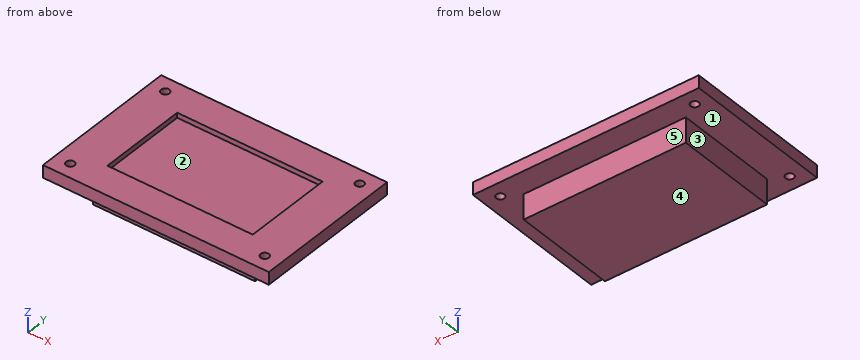
from build123d import *

# Parameters (mm, degrees)
F0_W     = 115
F0_H     = 76.2
F1_DEPTH = 6.35
F2_W     = 82.55
F2_H     = 52.3875
F3_DEPTH = 12.7
F4_W     = 74
F4_H     = 45
F5_DEPTH = 2.54
F7_D     = 4.1656


with BuildPart() as f1:
    # F0 (on Top) → F1 (new body)
    with BuildSketch(Plane.XY):
        with Locations((4.230735, 2.938756)):
            Rectangle(F0_W, F0_H)
    extrude(amount=F1_DEPTH)

    # F2 (on face) → F3 (join)
    with BuildSketch(Plane(origin=(0, 0, 0), x_dir=(1, 0, 0), z_dir=(0, 0, -1))):
        with Locations((4.225135, -2.716506)):
            Rectangle(F2_W, F2_H)
    extrude(amount=F3_DEPTH)

    # F4 (on face) → F5 (cut)
    with BuildSketch(Plane.XY.offset(6.35)):
        with Locations((4.228535, 2.943156)):
            Rectangle(F4_W, F4_H)
    extrude(amount=-F5_DEPTH, mode=Mode.SUBTRACT)

    # F7 (through all)
    with Locations(Plane.XY.offset(6.35)):
        with Locations((-45.269265, 33.538756), (53.730735, 33.538756), (53.730735, -27.668244), (-45.269265, -27.668244)):
            Hole(F7_D / 2)


solid = f1.part
For this review, take the finished solid that the model builds, in its own axes (mm). Face numbers are marked on the shaded views. A direction names the side the tool comes from. Coordinates: 2 decimals unless noted, no trailing zeros. Loops run counter-clockwise (first coordinate to the right, second up) from the corner with the lowest first, then second, coordinate; pieces in that order, holes last. Notation, with made-up numbers: (71, -25) - (111, -25) arc R24 cw to (111, -6) - close; hole circle Ø9 at (-33.5, -9). An arc over 180 degrees is marked (long way). Return JSON: item names as keys, results as strings.
Item 1: Take a section at C-C (z = -6.75). Give the boundary of the cut face in (x, y).
Determined:
{"outline": "(-37.05, -23.48) - (45.5, -23.48) - (45.5, 28.91) - (-37.05, 28.91) - close"}
Item 2: Take a section at B-B (x = 11). Give the boundary of the cut face in (y, z).
Determined:
{"outline": "(-35.16, 0) - (-23.48, 0) - (-23.48, -12.7) - (28.91, -12.7) - (28.91, 0) - (41.04, 0) - (41.04, 6.35) - (25.44, 6.35) - (25.44, 3.81) - (-19.56, 3.81) - (-19.56, 6.35) - (-35.16, 6.35) - close"}
Item 3: For the marked faces 4 and 5, list the 3-axis set-ups (+Z, -Z, +X, -X, +Y, -Y) from which the entire face can be reached by the end or side of a thin tool; tool diameter is ignored.
Determined:
{"face 4": "-Z, +X, -X, +Y, -Y", "face 5": "-Z, +X, -X, +Y"}
Item 4: Mouldability with a two-part tool opening along X and no side actions: class the marked faces 1, 2 and 3 as pulls with the +X half, pulls with the -X half, needs draft (parallel to the pull), parting line crosses it, or undercut.
Determined:
{"face 1": "needs draft", "face 2": "undercut", "face 3": "pulls with the -X half"}
Item 5: For line 1 (X direction, y = -15.5, z = 5.75); line 2 (Z direction, x = 40.5, y = 35.5); line 3 (Y direction, x = -1.5, z = -5), list the stretches that pass through material, from the lowest coordinate up.
Determined:
{"line 1": "x = -53.27 to -32.77, 41.23 to 61.73", "line 2": "z = 0 to 6.35", "line 3": "y = -23.48 to 28.91"}
Item 6: Take a section at A-A (y = 27). Give the boundary of the cut face in (x, z), then the cut area to 3 significant figures.
Determined:
{"outline": "(-53.27, 0) - (-37.05, 0) - (-37.05, -12.7) - (45.5, -12.7) - (45.5, 0) - (61.73, 0) - (61.73, 6.35) - (-53.27, 6.35) - close", "area": "1,780 mm2"}
Item 7: Take a section at D-D (y = -5). Give the boundary of the cut face in (x, z).
Determined:
{"outline": "(-53.27, 0) - (-37.05, 0) - (-37.05, -12.7) - (45.5, -12.7) - (45.5, 0) - (61.73, 0) - (61.73, 6.35) - (41.23, 6.35) - (41.23, 3.81) - (-32.77, 3.81) - (-32.77, 6.35) - (-53.27, 6.35) - close"}
Item 8: Insertion check: pin 1 (1.5 mm diameter, centred on x = 38.5, z = -8, fed in from +Y); pin 2 (10 mm diameter, centred on x = -19.5, z = -7, fed in from -Y); pin 3 (13.5 mm diameter, centred on x = -9.5, y = 6, fed in from +Z). Each pin has a flat end and moves straight along its axis. Give the tip position at first contact, or say it passes through.
Determined:
{"pin 1": "stops at y = 28.91", "pin 2": "stops at y = -23.48", "pin 3": "stops at z = 3.81"}
